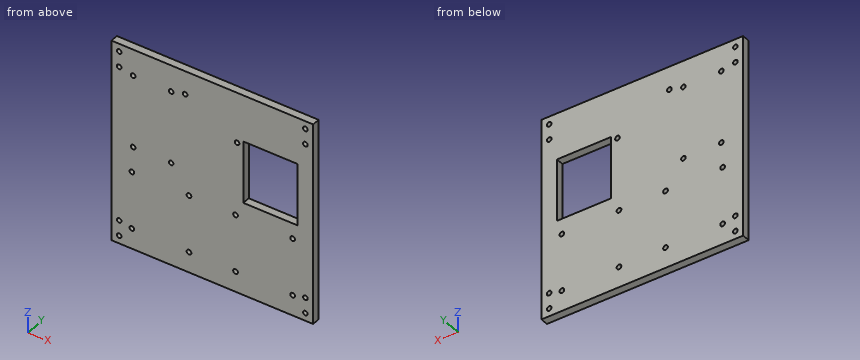
from build123d import *

# Parameters (mm, degrees)
SKETCH1_W           = 130
SKETCH1_H           = 130
BOSS_EXTRUDE1_DEPTH = 5
SKETCH4_R           = 1.5
CUT_EXTRUDE1_DEPTH  = 5
SKETCH8_R           = 1.5
CUT_EXTRUDE4_DEPTH  = 5
SKETCH9_W           = 35
SKETCH9_H           = 40
CUT_EXTRUDE5_DEPTH  = 5
SKETCH10_R          = 1.5
CUT_EXTRUDE6_DEPTH  = 5
SKETCH11_R          = 1.525
SKETCH11_R_2        = 1.5
CUT_EXTRUDE7_DEPTH  = 5
SKETCH12_R          = 1.5
CUT_EXTRUDE8_DEPTH  = 5


with BuildPart() as part:
    # Sketch1 → Boss-Extrude1 (new body)
    with BuildSketch(Plane(origin=(0, 0, 0), x_dir=(1, 0, 0), z_dir=(0, 1, 0))):
        Rectangle(SKETCH1_W, SKETCH1_H)
    extrude(amount=BOSS_EXTRUDE1_DEPTH)

    # Sketch4 → Cut-Extrude1 (cut)
    with BuildSketch(Plane(origin=(0, 5, 0), x_dir=(1, 0, 0), z_dir=(0, 1, 0))):
        with Locations(Location((60, 60, 0), (0, 0, 270))):
            Circle(SKETCH4_R)
        with Locations(Location((60, -60, 0), (0, 0, 270))):
            Circle(SKETCH4_R)
        with Locations(Location((-60, -60, 0), (0, 0, 270))):
            Circle(SKETCH4_R)
        with Locations(Location((-60, 60, 0), (0, 0, 270))):
            Circle(SKETCH4_R)
    extrude(amount=-CUT_EXTRUDE1_DEPTH, mode=Mode.SUBTRACT)

    # Sketch8 → Cut-Extrude4 (cut)
    with BuildSketch(Plane(origin=(0, 5, 0), x_dir=(1, 0, 0), z_dir=(0, 1, 0))):
        with Locations(Location((-60, 50, 0), (0, 0, 270))):
            Circle(SKETCH8_R)
        with Locations(Location((60, 50, 0), (0, 0, 270))):
            Circle(SKETCH8_R)
        with Locations(Location((60, -50, 0), (0, 0, 270))):
            Circle(SKETCH8_R)
        with Locations(Location((-60, -50, 0), (0, 0, 270))):
            Circle(SKETCH8_R)
    extrude(amount=-CUT_EXTRUDE4_DEPTH, mode=Mode.SUBTRACT)

    # Sketch9 → Cut-Extrude5 (cut)
    with BuildSketch(Plane(origin=(0, 5, 0), x_dir=(1, 0, 0), z_dir=(0, 1, 0))):
        with Locations((37.5, -15)):
            Rectangle(SKETCH9_W, SKETCH9_H)
    extrude(amount=-CUT_EXTRUDE5_DEPTH, mode=Mode.SUBTRACT)

    # Sketch10 → Cut-Extrude6 (cut)
    with BuildSketch(Plane(origin=(0, 5, 0), x_dir=(1, 0, 0), z_dir=(0, 1, 0))):
        with Locations(Location((-17.5, -50, 0), (0, 0, 270))):
            Circle(SKETCH10_R)
    extrude(amount=-CUT_EXTRUDE6_DEPTH, mode=Mode.SUBTRACT)

    # Sketch11 → Cut-Extrude7 (cut)
    with BuildSketch(Plane(origin=(0, 5, 0), x_dir=(1, 0, 0), z_dir=(0, 1, 0))):
        with Locations(Location((-51.803699422, 51.8, 0), (0, 0, 270))):
            Circle(SKETCH11_R)
        with Locations(Location((-14.996300578, 51.8, 0), (0, 0, 270))):
            Circle(SKETCH11_R)
        with Locations(Location((14.996300578, 51.8, 0), (0, 0, 270))):
            Circle(SKETCH11_R)
        with Locations(Location((51.803699422, 51.8, 0), (0, 0, 270))):
            Circle(SKETCH11_R)
        with Locations(Location((51.803699422, 14.95, 0), (0, 0, 270))):
            Circle(SKETCH11_R)
        with Locations(Location((14.996300578, 14.95, 0), (0, 0, 270))):
            Circle(SKETCH11_R)
        with Locations(Location((-14.996300578, 14.95, 0), (0, 0, 270))):
            Circle(SKETCH11_R)
        with Locations(Location((-51.803699422, 14.95, 0), (0, 0, 270))):
            Circle(SKETCH11_R)
        with Locations(Location((-51, -1.5, 0), (0, 0, 270))):
            Circle(SKETCH11_R_2)
        with Locations(Location((-26.5, -1.5, 0), (0, 0, 270))):
            Circle(SKETCH11_R_2)
        with Locations(Location((-26.5, -48, 0), (0, 0, 270))):
            Circle(SKETCH11_R_2)
        with Locations(Location((-51, -48, 0), (0, 0, 270))):
            Circle(SKETCH11_R_2)
    extrude(amount=-CUT_EXTRUDE7_DEPTH, mode=Mode.SUBTRACT)

    # Sketch12 → Cut-Extrude8 (cut)
    with BuildSketch(Plane(origin=(0, 5, 0), x_dir=(1, 0, 0), z_dir=(0, 1, 0))):
        with Locations(Location((16, -32.5, 0), (0, 0, 270))):
            Circle(SKETCH12_R)
    extrude(amount=-CUT_EXTRUDE8_DEPTH, mode=Mode.SUBTRACT)


solid = part.part
Geometry check sheet. Reference: the model listing, model coordinates, mm. Coordinates: 2 decimals unless noted, no trailing zeros. Write each loop counter-clockwise with the first axis right and the second up, starting at its lowest first coordinate (ties: lowest second). Pieces come first, ordered by that corner, then holes. Notation, with made-up numbers: (81.25, -23) -> (89.25, -23) arc R26 cw to (89.25, 14) -> close; hole circle Ø6 at (64.25, -13). An arc over 180 degrees is marked (long way). One line per question, with ' | ' between items.
1. Depth check by flat-ended pin: pin 1 Ø3.5 at (x, z) = (16, 32.5) entering from +Y. Enter the tip coordinate at first touch or a pass-through.
Answers:
pin 1: stops at y = 5
2. Cross-section at D-D on z = 18. Record the cut outline in (x, y), and give its area (3 significant figures).
Answers:
outline: (-65, 0) -> (20, 0) -> (20, 5) -> (-65, 5) -> close; (55, 0) -> (65, 0) -> (65, 5) -> (55, 5) -> close | area: 475 mm²
3. Cross-section at C-C on x = -26.5. Record the cut outline in (y, z), and give its area (3 significant figures).
Answers:
outline: (0, -65) -> (5, -65) -> (5, 0) -> (0, 0) -> close; (0, 3) -> (5, 3) -> (5, 46.5) -> (0, 46.5) -> close; (0, 49.5) -> (5, 49.5) -> (5, 65) -> (0, 65) -> close | area: 620 mm²
4. Cross-section at B-B on z = 32.5. Record the cut outline in (x, y).
Answers:
outline: (-65, 0) -> (14.5, 0) -> (14.5, 5) -> (-65, 5) -> close; (17.5, 0) -> (20, 0) -> (20, 5) -> (17.5, 5) -> close; (55, 0) -> (65, 0) -> (65, 5) -> (55, 5) -> close
5. Cross-section at A-A on x = 60. Record the cut outline in (y, z), and give its area (3 significant figures).
Answers:
outline: (0, -65) -> (5, -65) -> (5, -61.5) -> (0, -61.5) -> close; (0, -58.5) -> (5, -58.5) -> (5, -51.5) -> (0, -51.5) -> close; (0, -48.5) -> (5, -48.5) -> (5, 48.5) -> (0, 48.5) -> close; (0, 51.5) -> (5, 51.5) -> (5, 58.5) -> (0, 58.5) -> close; (0, 61.5) -> (5, 61.5) -> (5, 65) -> (0, 65) -> close | area: 590 mm²
6. Thickness scan on probe 1 along X at (y, z) = (4, -51.8); probe 2 along X at (y, z) = (2.75, 50); probe 3 along X at (y, z) = (4.2, 32.5). Record the ranges inside material, lowest first. Write a range as from..to.
Answers:
probe 1: x = -65..-53.33, -50.28..-16.52, -13.47..13.47, 16.52..50.28, 53.33..65 | probe 2: x = -65..-61.5, -58.5..-19, -16..58.5, 61.5..65 | probe 3: x = -65..14.5, 17.5..20, 55..65
